Can you work these out from the model? Positions are in its coordinate system, mm. Face numbers are marked on the shaded views. Coordinates: 2 decimals unless noted, no trailing zeros. Order: outer loops, then holes, each group sorted by start corner. A loop starts at its lowest first (then second) coordinate and runs counter-clockwise, first axis right, second up. Notation, with made-up numbers: (-39, -11.75) -> (4, -11.75) arc R4 cw to (4, -6.75) -> close; hole circle Ø10 at (76, 33). An arc over 180 degrees is marked (long way). Answer in a Markdown table with one row per item.
```python
from build123d import *

# Parameters (mm, degrees)
SKETCH1_W           = 25.4
SKETCH1_H           = 25.4
BOSS_EXTRUDE1_DEPTH = 38.1
SKETCH3_R           = 3.175
CUT_EXTRUDE1_DEPTH  = 12.7
SKETCH2_R           = 3.175
CUT_EXTRUDE2_DEPTH  = 48.519048812


with BuildPart() as part:
    # Sketch1 → Boss-Extrude1 (new body)
    with BuildSketch(Plane.XY):
        Rectangle(SKETCH1_W, SKETCH1_H)
    extrude(amount=BOSS_EXTRUDE1_DEPTH)

    # Sketch3 → Cut-Extrude1 (cut)
    with BuildSketch(Plane.XY.offset(38.1)):
        Circle(SKETCH3_R)
    extrude(amount=-CUT_EXTRUDE1_DEPTH, mode=Mode.SUBTRACT)

    # Sketch2 → Cut-Extrude2 (cut, through all)
    with BuildSketch(Plane.ZY.offset(12.7)):
        with Locations((19.05, -1.905)):
            Circle(SKETCH2_R)
    extrude(amount=-CUT_EXTRUDE2_DEPTH, mode=Mode.SUBTRACT)


solid = part.part
```
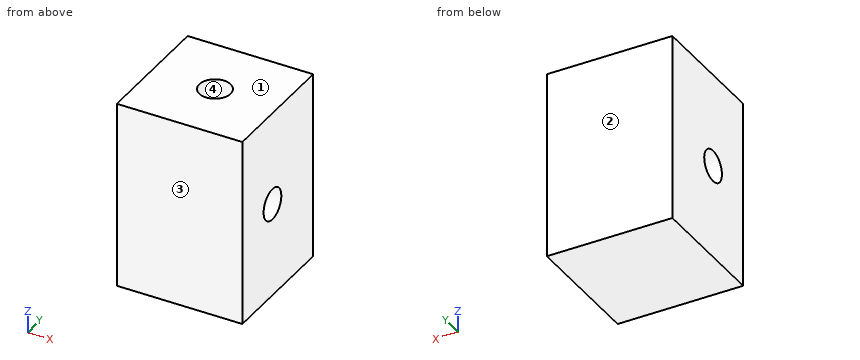
(1) Will this pin go through, and if not, where does the flat tip stop? pin 1 Ø3 at (x, y) = (1.5, 0.5) entering from +Z.
Response values:
| item | result |
|---|---|
| pin 1 | z = 25.4 |
(2) Suppose I cut it at D-D (x = 0.75). Please give me the cut outline in (y, z) (3 decimals), and give its area (3 significant figures).
Response values:
| item | result |
|---|---|
| outline | (-12.7, 0) -> (12.7, 0) -> (12.7, 38.1) -> (3.085, 38.1) -> (3.085, 25.4) -> (-3.085, 25.4) -> (-3.085, 38.1) -> (-12.7, 38.1) -> close; hole circle Ø6.35 at (-1.905, 19.05) |
| area | 858 mm2 |
(3) Suppose I cut it at A-A (z = 19.05). Please give me the cut outline in (x, y), and give its area (3 significant figures).
Response values:
| item | result |
|---|---|
| outline | (-12.7, -12.7) -> (12.7, -12.7) -> (12.7, -5.08) -> (-12.7, -5.08) -> close; (-12.7, 1.27) -> (12.7, 1.27) -> (12.7, 12.7) -> (-12.7, 12.7) -> close |
| area | 484 mm2 |
(4) Suppose I cut it at C-C (z = 34). Please give me the cut outline in (x, y) (3 decimals).
Response values:
| item | result |
|---|---|
| outline | (-12.7, -12.7) -> (12.7, -12.7) -> (12.7, 12.7) -> (-12.7, 12.7) -> close; hole circle Ø6.35 at (0, 0) |
(5) We'd pull the mould along Y, two halves only. Please class the marked faces 1, 2, 3 and 4: +Y half, -Y half, draft (parallel to the pull), parting line (faces both ways), or undercut.
Response values:
| item | result |
|---|---|
| face 1 | draft |
| face 2 | +Y half |
| face 3 | -Y half |
| face 4 | undercut |
(6) I need wall thicknesses on line 1 (Y direction, x = 7.25, z = 19.05); line 2 (Z direction, x = -5.75, y = -2); line 3 (Y direction, x = 0, z = 34.5) (3 decimals). Which ranges of each line are inside material? Lowest first, please. Write a range as [from, to].
Response values:
| item | result |
|---|---|
| line 1 | [-12.7, -5.08], [1.27, 12.7] |
| line 2 | [0, 15.88], [22.22, 38.1] |
| line 3 | [-12.7, -3.175], [3.175, 12.7] |
(7) Suppose I cut it at B-B (y = 0). Please give me the cut outline in (x, z) (3 decimals), and give its area (3 significant figures).
Response values:
| item | result |
|---|---|
| outline | (-12.7, 0) -> (12.7, 0) -> (12.7, 16.51) -> (-12.7, 16.51) -> close; (-12.7, 21.59) -> (12.7, 21.59) -> (12.7, 38.1) -> (3.175, 38.1) -> (3.175, 25.4) -> (-3.175, 25.4) -> (-3.175, 38.1) -> (-12.7, 38.1) -> close |
| area | 758 mm2 |
